```python
from build123d import *

# Parameters (mm, degrees)
BOSS_EXTRUDE1_DEPTH = 50.8
BOSS_EXTRUDE2_DEPTH = 6.35
SKETCH3_R           = 2.0193
CUT_EXTRUDE1_DEPTH  = 61.017858453
SKETCH4_R           = 2.6289
CUT_EXTRUDE2_DEPTH  = 57.954059175


with BuildPart() as part:
    # Sketch1 → Boss-Extrude1 (new body)
    with BuildSketch(Plane(origin=(0, 0, 0), x_dir=(1, 0, 0), z_dir=(0, 1, 0))):
        Polygon((7.332348419, 12.7), (-7.332348419, 12.7), (-14.664696837, 0), (-7.332348419, -12.7), (7.332348419, -12.7), (14.664696837, 0), align=None)
        Polygon((3.717500648, 6.4389), (-3.717500648, 6.4389), (-7.435001297, 0), (-3.717500648, -6.4389), (3.717500648, -6.4389), (7.435001297, 0), align=None, mode=Mode.SUBTRACT)
    extrude(amount=BOSS_EXTRUDE1_DEPTH)

    # Sketch2 → Boss-Extrude2 (add)
    with BuildSketch(Plane.XZ):
        Polygon((3.717500648, -6.4389), (-3.717500648, -6.4389), (-7.435001297, 0), (-3.717500648, 6.4389), (3.717500648, 6.4389), (7.435001297, 0), align=None)
    extrude(amount=-BOSS_EXTRUDE2_DEPTH)

    # Sketch3 → Cut-Extrude1 (cut, through all)
    with BuildSketch(Plane(origin=(10.998522628, 0, 6.35), x_dir=(0.5000000000000001, 0, -0.8660254037844386), z_dir=(0.8660254037844386, 0, 0.5000000000000001))):
        with Locations((0, 19.05)):
            Circle(SKETCH3_R)
        with Locations((0, 38.1)):
            Circle(SKETCH3_R)
    extrude(amount=-CUT_EXTRUDE1_DEPTH, mode=Mode.SUBTRACT)

    # Sketch4 → Cut-Extrude2 (cut, through all)
    with BuildSketch(Plane(origin=(-5.576250972, 0, -3.21945), x_dir=(0.49999999999999967, 0, -0.8660254037844388), z_dir=(0.8660254037844388, 0, 0.49999999999999967))):
        with Locations((0, 38.1)):
            Circle(SKETCH4_R)
        with Locations((0, 19.05)):
            Circle(SKETCH4_R)
    extrude(amount=-CUT_EXTRUDE2_DEPTH, mode=Mode.SUBTRACT)


solid = part.part
```
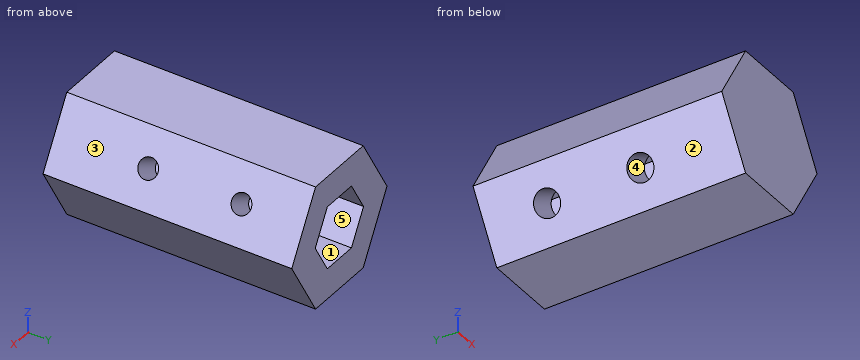
Verification items for the finished model (mm, model axes). Face numbers are marked on the shaded views. A direction names the side the tool comes from. Give positions to 0.01 mm unless a question says otherwise; leave off trailing zeros. Loops run counter-clockwise (first coordinate to the right, second up) from the corner with the lowest first, then second, coordinate; pieces in that order, holes last.
1. Set-up check for the marked faces 4 and 5: record each of +Z, -Z, +X, -X, +Y, -Y from which the full face is reachable in a straight line by a thin tool's end or side.
2. Go/stop test with flat-tipped pins: pin 1 Ø4 at (x, y) = (-10, 9) entering from -Z; pin 2 Ø6 at (y, z) = (6.5, 9) entering from +X; pin 3 Ø1.5 at (y, z) = (35, 2.5) entering from -X. Record where each tip stops, or that it passes through.
3. Mould release check, pull along X, two halves, no side actions. Record for the marked faces 1, 2 and 3: released by +X, released by -X, zero draft, split by the parting line, or undercut.
4. Thickness scan on line 1 (Z direction, x = -1.75, y = 31); line 2 (X direction, y = 27.5, z = -1.75); line 3 (Y direction, x = -6, z = -1.5). Record the ranges inside material, lowest first.
5. Section check C-C, the plane z = 0.75. Enter the section's corners in (x, y), then the cut area to 3 significant figures.
6. Section check B-B, the plane x = -0.5. Enter the section's corners in (y, z).
7. Section check D-D, the plane z = -4.25. Count the separate pieces of the cut face and the enclosed holes in it, then the cut area to 3 significant figures.
8. Section check A-A, the plane y = 42. Enter the section's corners in (x, z) (1 decimal).
Geometry says:
1. face 4: none
1. face 5: +Y
2. pin 1: stops at z = -11.54
2. pin 2: stops at x = 11.2
2. pin 3: stops at x = -13.65
3. face 1: undercut
3. face 2: released by -X
3. face 3: released by +X
4. line 1: z = -12.7 to -6.44, 6.44 to 12.7
4. line 2: x = -13.65 to -6.42, 6.42 to 13.65
4. line 3: y = 0 to 6.35
5. outline: (-14.23, 0) - (14.23, 0) - (14.23, 50.8) - (7, 50.8) - (7, 6.35) - (-7, 6.35) - (-7, 50.8) - (-14.23, 50.8) - close
5. area: 823 mm2
6. outline: (0, -12.7) - (50.8, -12.7) - (50.8, -6.44) - (6.35, -6.44) - (6.35, 6.44) - (50.8, 6.44) - (50.8, 12.7) - (0, 12.7) - close
7. separate pieces: 3
7. enclosed holes: 0
7. area: 731 mm2
8. outline: (-14.7, 0) - (-7.3, -12.7) - (7.3, -12.7) - (14.7, 0) - (7.3, 12.7) - (-7.3, 12.7) - close; hole (-7.4, 0) - (-3.7, -6.4) - (3.7, -6.4) - (7.4, 0) - (3.7, 6.4) - (-3.7, 6.4) - close
